The model under review builds one solid part; all positions refer to its coordinate system, in mm. A direction names the side the tool comes from. Coordinates: 2 decimals unless noted, no trailing zeros. Loops run counter-clockwise (first coordinate to the right, second up) from the corner with the lowest first, then second, coordinate; pieces in that order, holes last. Notation, with made-up numbers: (17.25, 7) -> (67.25, 7) arc R17 ccw to (67.25, 22) -> close; hole circle Ø3 at (60, -32). An arc over 180 degrees is marked (long way). One line per question, with ' | ' between items. Start each with the question number.
from build123d import *

# Parameters (mm, degrees)
SKETCH1_R           = 4.4
SKETCH1_R_2         = 4.2
SKETCH1_R_3         = 3.8
BOSS_EXTRUDE2_DEPTH = 1.778
SKETCH1_4_R         = 4.2
SKETCH1_4_R_2       = 3
SKETCH1_4_R_3       = 4.4
SKETCH1_4_R_4       = 3.175
SKETCH1_4_R_5       = 3.8
SKETCH1_4_R_6       = 2.8448
BOSS_EXTRUDE3_DEPTH = 4.953


with BuildPart() as part:
    # Sketch1 → Boss-Extrude2 (new body)
    with BuildSketch(Plane(origin=(0, 0, 0), x_dir=(1, 0, 0), z_dir=(0, 1, 0))):
        Polygon((-42.232830982, -41.594410903), (-33.088830982, -41.594410903), (-33.088830982, -47.944410903), (34.983169018, -47.944410903), (34.983169018, -41.594410903), (44.127169018, -41.594410903), (44.127169018, 66.863589097), (43.365169018, 66.863589097), (28.125169018, 66.863589097), (28.125169018, 75.499589097), (-26.992830982, 75.499589097), (-26.992830982, 66.863589097), (-42.232830982, 66.863589097), align=None)
        with Locations(Location((-27.642783289, -37.764613693, 0), (0, 0, 270))):
            Circle(SKETCH1_R, mode=Mode.SUBTRACT)
        with Locations(Location((29.507278107, -37.764613693, 0), (0, 0, 270))):
            Circle(SKETCH1_R, mode=Mode.SUBTRACT)
        with Locations(Location((-27.731568772, 19.395386307, 0), (0, 0, 270))):
            Circle(SKETCH1_R, mode=Mode.SUBTRACT)
        with Locations(Location((-17.958983642, 30.494821479, 0), (0, 0, 270))):
            Circle(SKETCH1_R_2, mode=Mode.SUBTRACT)
        with Locations(Location((-17.958983642, 47.403601479, 0), (0, 0, 270))):
            Circle(SKETCH1_R_2, mode=Mode.SUBTRACT)
        with Locations(Location((-8.7905296, 71.432825816, 0), (0, 0, 270))):
            Circle(SKETCH1_R_3, mode=Mode.SUBTRACT)
        with Locations(Location((29.428492634, 19.395386307, 0), (0, 0, 270))):
            Circle(SKETCH1_R, mode=Mode.SUBTRACT)
        with Locations(Location((35.241316358, 30.494821479, 0), (0, 0, 270))):
            Circle(SKETCH1_R_2, mode=Mode.SUBTRACT)
        with Locations(Location((20.4194704, 58.732825816, 0), (0, 0, 270))):
            Circle(SKETCH1_R_3, mode=Mode.SUBTRACT)
        with Locations(Location((35.241316358, 47.403601479, 0), (0, 0, 270))):
            Circle(SKETCH1_R_2, mode=Mode.SUBTRACT)
    extrude(amount=BOSS_EXTRUDE2_DEPTH)

    # Sketch1<4> → Boss-Extrude3 (add)
    # profile 1 of 10: a face of its own
    with BuildSketch(Plane(origin=(0, 0, 0), x_dir=(1, 0, 0), z_dir=(0, 1, 0))):
        with Locations(Location((-17.958983642, 47.403601479, 0), (0, 0, 270))):
            Circle(SKETCH1_4_R)
        with Locations(Location((-17.958983642, 47.403601479, 0), (0, 0, 270))):
            Circle(SKETCH1_4_R_2, mode=Mode.SUBTRACT)
    # profile 2 of 10: a face of its own
    with BuildSketch(Plane(origin=(0, 0, 0), x_dir=(1, 0, 0), z_dir=(0, 1, 0))):
        with Locations(Location((-17.958983642, 30.494821479, 0), (0, 0, 270))):
            Circle(SKETCH1_4_R)
        with Locations(Location((-17.958983642, 30.494821479, 0), (0, 0, 270))):
            Circle(SKETCH1_4_R_2, mode=Mode.SUBTRACT)
    # profile 3 of 10: a face of its own
    with BuildSketch(Plane(origin=(0, 0, 0), x_dir=(1, 0, 0), z_dir=(0, 1, 0))):
        with Locations(Location((35.241316358, 47.403601479, 0), (0, 0, 270))):
            Circle(SKETCH1_4_R)
        with Locations(Location((35.241316358, 47.403601479, 0), (0, 0, 270))):
            Circle(SKETCH1_4_R_2, mode=Mode.SUBTRACT)
    # profile 4 of 10: a face of its own
    with BuildSketch(Plane(origin=(0, 0, 0), x_dir=(1, 0, 0), z_dir=(0, 1, 0))):
        with Locations(Location((35.241316358, 30.494821479, 0), (0, 0, 270))):
            Circle(SKETCH1_4_R)
        with Locations(Location((35.241316358, 30.494821479, 0), (0, 0, 270))):
            Circle(SKETCH1_4_R_2, mode=Mode.SUBTRACT)
    # profile 5 of 10: a face of its own
    with BuildSketch(Plane(origin=(0, 0, 0), x_dir=(1, 0, 0), z_dir=(0, 1, 0))):
        with Locations(Location((-27.731568772, 19.395386307, 0), (0, 0, 270))):
            Circle(SKETCH1_4_R_3)
        with Locations(Location((-27.731568772, 19.395386307, 0), (0, 0, 270))):
            Circle(SKETCH1_4_R_4, mode=Mode.SUBTRACT)
    # profile 6 of 10: a face of its own
    with BuildSketch(Plane(origin=(0, 0, 0), x_dir=(1, 0, 0), z_dir=(0, 1, 0))):
        with Locations(Location((-27.642783289, -37.764613693, 0), (0, 0, 270))):
            Circle(SKETCH1_4_R_3)
        with Locations(Location((-27.642783289, -37.764613693, 0), (0, 0, 270))):
            Circle(SKETCH1_4_R_4, mode=Mode.SUBTRACT)
    # profile 7 of 10: a face of its own
    with BuildSketch(Plane(origin=(0, 0, 0), x_dir=(1, 0, 0), z_dir=(0, 1, 0))):
        with Locations(Location((29.507278107, -37.764613693, 0), (0, 0, 270))):
            Circle(SKETCH1_4_R_3)
        with Locations(Location((29.507278107, -37.764613693, 0), (0, 0, 270))):
            Circle(SKETCH1_4_R_4, mode=Mode.SUBTRACT)
    # profile 8 of 10: a face of its own
    with BuildSketch(Plane(origin=(0, 0, 0), x_dir=(1, 0, 0), z_dir=(0, 1, 0))):
        with Locations(Location((29.428492634, 19.395386307, 0), (0, 0, 270))):
            Circle(SKETCH1_4_R_3)
        with Locations(Location((29.428492634, 19.395386307, 0), (0, 0, 270))):
            Circle(SKETCH1_4_R_4, mode=Mode.SUBTRACT)
    # profile 9 of 10: a face of its own
    with BuildSketch(Plane(origin=(0, 0, 0), x_dir=(1, 0, 0), z_dir=(0, 1, 0))):
        with Locations(Location((-8.7905296, 71.432825816, 0), (0, 0, 270))):
            Circle(SKETCH1_4_R_5)
        with Locations(Location((-8.7905296, 71.432825816, 0), (0, 0, 270))):
            Circle(SKETCH1_4_R_6, mode=Mode.SUBTRACT)
    # profile 10 of 10: a face of its own
    with BuildSketch(Plane(origin=(0, 0, 0), x_dir=(1, 0, 0), z_dir=(0, 1, 0))):
        with Locations(Location((20.4194704, 58.732825816, 0), (0, 0, 270))):
            Circle(SKETCH1_4_R_5)
        with Locations(Location((20.4194704, 58.732825816, 0), (0, 0, 270))):
            Circle(SKETCH1_4_R_6, mode=Mode.SUBTRACT)
    extrude(amount=BOSS_EXTRUDE3_DEPTH)


solid = part.part
1) Machinability: for faces 1 (the face through (-16.697, 3.343, -43.398)), 2 (the face through (32.5, 4.953, -28.7)), which of the approach directions +Z, -Z, +X, -X, +Y, -Y give a long, thin tool a straight path to every point of the face, cutting with its end or side? Answer none if there is none.
2) Consider section A-A, the plane y = 4.1. Give the number of separate pieces and of enclosed holes in the cut face, plus the area to 3 significant figures.
3) Consider section B-B, the plane x = -10. Write out the cut boundary in (y, z).
4) Consider section C-C, the plane z = 26.5. Write out the cut boundary in (x, y).
5) Insertion check: pin 1 Ø5.5 at (x, z) = (-27.73, -19.4) entering from -Y; pin 2 Ø10 at (x, z) = (-32.5, -42.5) entering from +Y; pin 3 Ø0.9 at (x, y) = (-32, 1) entering from -Z; pin 4 Ø0.5 at (x, y) = (-35.5, 1) entering from +Z. Each pin has a flat end and moves straight along its axis. Give the tip position at first contact, or say it passes through.
6) Mouldability with a two-part tool opening along X and no side actions: class faces 3 (the face through (18.11, 3.34, -61.75)), 4 (the face through (33, 4.953, -45)), 5 (the face through (19.33, 2.442, -56.105)) as +X half, -X half, draft (parallel to the pull), parting line (faces both ways), or undercut.
7) Wall thickness on L1, parallel to X at y = 1.5, z = -29.5; L2, parallel to X at y = 1.55, z = -48.5; L3, parallel to Z at x = -33.5, y = 1.55: over which ranges is each line inside the solid? List them lowest first.
Filled sheet:
1) face 1: +Y | face 2: +Z, -Z, +X, -X, +Y
2) separate pieces: 10 | enclosed holes: 10 | area: 265 mm^2
3) outline: (0, -75.5) -> (1.78, -75.5) -> (1.78, -75.04) -> (4.95, -75.04) -> (4.95, -74.01) -> (0, -74.01) -> close; (0, -68.86) -> (4.95, -68.86) -> (4.95, -67.83) -> (1.78, -67.83) -> (1.78, 47.94) -> (0, 47.94) -> close
4) outline: (-42.23, 0) -> (44.13, 0) -> (44.13, 1.78) -> (-42.23, 1.78) -> close
5) pin 1: through | pin 2: y = 1.78 | pin 3: z = -66.86 | pin 4: z = 41.59
6) face 3: parting line | face 4: draft | face 5: undercut
7) L1: -42.23 to -20.79, -15.13 to 32.41, 38.07 to 44.13 | L2: -42.23 to -20.75, -15.17 to 32.45, 38.03 to 44.13 | L3: -66.86 to 41.59
